Design review of the part built by this model. Coordinates are the model's own, in mm. Face numbers are marked on the shaded views. A direction names the side the tool comes from. Round coordinates to 2 decimals unless told otherwise and drop trailing zeros. Order: outer loops, then holes, each group sorted by start corner. A loop starts at its lowest first (then second) coordinate and runs counter-clockwise, first axis right, second up. Notation, with made-up numbers: M 58.5,-35 L 106.5,-35 A32 ccw 106.5,-3 Z; hole C 45,68.5 d6. An arc over 180 degrees is marked long. Use a Markdown table: item, result. Add a question column.
(1) To check wall thickness, follow probe 1 along Y at (x, z) = (-18, 111); probe 2 along Z at (x, y) = (-1.5, 2.5); probe 3 along X at (y, z) = (-0.5, 83). State the ranges of each line that lie inside material, in increasing order. Write a range as from..to.
(2) Take a section at A-A (y = 4.25). Write out the cut boundary in (x, z).
(3) For pin 1 (6 mm diameter, centred on x = -20.5, z = 105, fed in from +Y); pin 2 (5 mm diameter, centred on y = 0.5, z = 79, fed in from +X); pin 3 (0.7 mm diameter, centred on x = -0.07, y = 6.14, fed in from +Z); pin 4 (1.8 mm diameter, centred on y = 0, z = -1, fed in from +X), all flat-tipped, find the tip position at first contact; note any pin that passes through.
(4) Take a section at B-B (x = -9). Write out the cut boundary in (y, z).
(5) Machinability: for the marked faces 1 and 2, which of the approach directions +Z, -Z, +X, -X, +Y, -Y give a long, thin tool a straight path to every point of the face, cutting with its end or side? Answer none if there is none.
Autodesk Inventor part; units mm, degrees
ref_plane "YZ Plane" through (0, 0, 0) normal (1, 0, 0) x (0, 1, 0)
ref_plane "XZ Plane" through (0, 0, 0) normal (0, 1, 0) x (-1, 0, 0)
ref_plane "XY Plane" through (0, 0, 0) normal (0, 0, 1) x (1, 0, 0)
sketch "Sketch1" plane through (0, 0, 0) normal (0, 0, 1) x (1, 0, 0)
  line L0 (-6.698639, 7.691729) -> (4.001361, 7.691729)
  line L1 (4.001361, 7.691729) -> (4.001361, -6.308271)
  line L2 (4.001361, -6.308271) -> (-6.698639, -6.308271)
  line L3 (-6.698639, -6.308271) -> (-6.698639, 7.691729)
  line L4 (4.001361, -6.308271) -> (-6.698639, -6.308271)
  line L5 (-6.698639, -6.308271) -> (-6.698639, -2.808271)
  line L6 (-6.698639, -2.808271) -> (4.001361, -2.808271)
  line L7 (4.001361, -2.808271) -> (4.001361, -6.308271)
  line L8 (-6.698639, -6.308271) -> (-5.698639, -6.308271)
  line L9 (-5.698639, -6.308271) -> (-5.698639, 7.691729)
  line L10 (-5.698639, 7.691729) -> (-6.698639, 7.691729)
  line L11 (-6.698639, 7.691729) -> (-6.698639, -6.308271)
  line L12 (-5.698639, -2.808271) -> (3.472299, -2.808271)
  line L13 (3.472299, -2.808271) -> (3.472299, -0.408271)
  line L14 (3.472299, -0.408271) -> (-5.698639, -0.408271)
  line L15 (-5.698639, -0.408271) -> (-5.698639, -2.808271)
  line L16 (-5.698639, -0.408271) -> (-1.298639, -0.408271)
  line L17 (-1.298639, -0.408271) -> (-1.298639, -2.808271)
  line L18 (-1.298639, -2.808271) -> (-5.698639, -2.808271)
  line L19 (-5.698639, -2.808271) -> (-5.698639, -0.408271)
  point P0 (0, 0)
  dimension "d0" = 10.7
  dimension "d1" = 14
  dimension "d2" = 3.5
  dimension "d3" = 1
  dimension "d4" = 2.4
  dimension "d5" = 4.4
extrude "Extrusion1" add sketch "Sketch1" against normal blind 1.6
extrude "Extrusion2" add sketch "Sketch1" along normal blind 1.1 contours L14 L17 L6 L9
sketch "Sketch2" plane through (0, 0, 0) normal (0, 0, 1) x (1, 0, 0)
  line L0 (-1.298639, -0.408271) -> (-1.298639, -2.808271)
  line L1 (-1.298639, -2.808271) -> (-5.698639, -2.808271)
  line L2 (-5.698639, -2.808271) -> (-5.698639, -0.408271)
  line L3 (-5.698639, -0.408271) -> (-1.298639, -0.408271)
  line L4 (4.001361, 7.691729) -> (-6.698639, 7.691729)
  line L5 (-6.698639, 7.691729) -> (-6.698639, -6.308271)
  line L6 (-6.698639, -6.308271) -> (4.001361, -6.308271)
  line L7 (4.001361, -6.308271) -> (4.001361, 7.691729)
  line L8 (4.001361, -6.308271) -> (4.001361, 7.691729)
  line L9 (-6.698639, 7.691729) -> (-6.698639, -6.308271)
  line L10 (4.001361, -6.308271) -> (-6.698639, -6.308271)
  line L11 (-6.698639, -6.308271) -> (-6.698639, -5.308271)
  line L12 (-6.698639, -5.308271) -> (4.001361, -5.308271)
  line L13 (4.001361, -5.308271) -> (4.001361, -6.308271)
  line L14 (4.001361, -6.308271) -> (3.001361, -6.308271)
  line L15 (3.001361, -6.308271) -> (3.001361, -2.808271)
  line L16 (3.001361, -2.808271) -> (4.001361, -2.808271)
  line L17 (4.001361, -2.808271) -> (4.001361, -6.308271)
  line L18 (-6.698639, -6.308271) -> (-0.098639, -6.308271)
  line L19 (-0.098639, -6.308271) -> (-0.098639, -2.808271)
  line L20 (-0.098639, -2.808271) -> (-6.698639, -2.808271)
  line L21 (-6.698639, -2.808271) -> (-6.698639, -6.308271)
  circle A0 centre (1.451361, -3.758271) radius 1.55
  point P0 (0, 0)
  dimension "d10" = 1
  dimension "d11" = 1
  dimension "d12" = 6.6
extrude "Extrusion3" cut sketch "Sketch2" against normal through all contours A0
sketch "Sketch3" plane through (0, 0, 0) normal (0, 0, 1) x (1, 0, 0)
  line L0 (4.001361, 7.691729) -> (4.001361, -6.308271)
  line L1 (-6.698639, 7.691729) -> (4.001361, 7.691729)
  line L2 (4.001361, 7.691729) -> (4.001361, 6.691729)
  line L3 (4.001361, 6.691729) -> (-6.698639, 6.691729)
  line L4 (-6.698639, 6.691729) -> (-6.698639, 7.691729)
  line L5 (-6.698639, 7.691729) -> (-5.698639, 7.691729)
  line L6 (-5.698639, 7.691729) -> (-5.698639, 5.612457)
  line L7 (-5.698639, 5.612457) -> (-6.698639, 5.612457)
  line L8 (-6.698639, 5.612457) -> (-6.698639, 7.691729)
  line L9 (-5.698639, 6.691729) -> (-4.598639, 6.691729)
  line L10 (-4.598639, 6.691729) -> (-4.598639, 6.161753)
  line L11 (-4.598639, 6.161753) -> (-5.698639, 6.161753)
  line L12 (-5.698639, 6.161753) -> (-5.698639, 6.691729)
  circle A0 centre (-5.148639, 6.141729) radius 0.55
  circle A1 centre (-2.608639, 6.141729) radius 0.55
  line L13 (-2.058639, 6.161753) -> (-3.158639, 6.161753)
  circle A2 centre (-0.068639, 6.141729) radius 0.55
  line L14 (0.481361, 6.161753) -> (-0.618639, 6.161753)
  circle A3 centre (2.471361, 6.141729) radius 0.55
  line L15 (3.021361, 6.161753) -> (1.921361, 6.161753)
  circle A4 centre (1.451361, -3.758271) radius 1.55
  line L16 (-1.298639, -0.408271) -> (-1.298639, -2.808271)
  line L17 (-1.298639, -2.808271) -> (-5.698639, -2.808271)
  line L18 (-5.698639, -2.808271) -> (-5.698639, -0.408271)
  line L19 (-5.698639, -0.408271) -> (-1.298639, -0.408271)
  line L20 (4.001361, 7.691729) -> (-6.698639, 7.691729)
  line L21 (-6.698639, 7.691729) -> (-6.698639, -6.308271)
  line L22 (-6.698639, -6.308271) -> (4.001361, -6.308271)
  line L23 (4.001361, -6.308271) -> (4.001361, 7.691729)
  line L24 (-6.698639, -6.308271) -> (-5.698639, -6.308271)
  line L25 (-5.698639, -6.308271) -> (-5.698639, -3.371834)
  line L26 (-5.698639, -3.371834) -> (-6.698639, -3.371834)
  line L27 (-6.698639, -3.371834) -> (-6.698639, -6.308271)
  line L28 (-6.698639, -6.308271) -> (4.001361, -6.308271)
  line L29 (-6.698639, -6.308271) -> (-3.498639, -6.308271)
  line L30 (-3.498639, -6.308271) -> (-3.498639, -5.308271)
  line L31 (-3.498639, -5.308271) -> (-6.698639, -5.308271)
  line L32 (-6.698639, -5.308271) -> (-6.698639, -6.308271)
  line L33 (-5.698639, -6.308271) -> (-4.598639, -6.308271)
  line L34 (-4.598639, -6.308271) -> (-4.598639, -3.371834)
  line L35 (-4.598639, -3.371834) -> (-5.698639, -3.371834)
  line L36 (-5.698639, -3.371834) -> (-5.698639, -6.308271)
  circle A5 centre (-5.148639, -4.758271) radius 0.55
  circle A6 centre (-2.608639, -4.758271) radius 0.55
  line L37 (-0.958639, -5.308271) -> (-4.158639, -5.308271)
  point P0 (0, 0)
  dimension "d15" = 1
  dimension "d16" = 1
  dimension "d17" = 1.1
  dimension "d20" = 2.54
  dimension "d25" = 1
  dimension "d26" = 1
  dimension "d27" = 1.1
  dimension "d30" = 2.54
sketch "Sketch3 outline for Extrusion4" plane through (0, 0, 0) normal (0, 0, 1) x (1, 0, 0)
  circle A0 centre (-5.148639, -4.758271) radius 0.55
  circle A1 centre (-2.608639, -4.758271) radius 0.55
  circle A2 centre (2.471361, 6.141729) radius 0.55
  circle A3 centre (-0.068639, 6.141729) radius 0.55
  circle A4 centre (-2.608639, 6.141729) radius 0.55
  circle A5 centre (-5.148639, 6.141729) radius 0.55
extrude "Extrusion4" cut sketch "Sketch3 outline for Extrusion4" against normal through all
sketch "Sketch4" plane through (-5.698639, -0.408271, 0) normal (0, 1, 0) x (1, 0, 0)
  line L0 (0, 0) -> (4.4, 0)
  line L1 (0, 0) -> (0, -1.1)
  line L2 (4.4, -1.1) -> (0, -1.1)
  line L3 (4.4, 0) -> (4.4, -1.1)
  line L4 (0, -1.1) -> (4.4, -1.1)
  line L5 (2.2, -1.1) -> (2.2, 3.167795)
  line L6 (0, -1.1) -> (-26.909589, -122.481313)
  line L7 (0, -1.1) -> (4.299042, 18.291726)
  line L8 (4.4, -1.1) -> (31.309589, -122.481313)
  line L9 (4.4, -1.1) -> (0.100958, 18.291726)
  circle A0 centre (2.2, 8.823559) radius 134.49289
  point P0 (5.698639, 0)
  dimension "d37" = 12.5
extrude "Extrusion5" add sketch "Sketch4" against normal up to surface (2.4 mm away) contours L2 L8 A0 L6
sketch "Sketch5" plane through (-5.698639, -0.408271, 1.1) normal (-0.976296, 0, -0.2164396) x (-0.2164396, 0, 0.976296)
  line L0 (0, -2.4) -> (124.328392, -2.4)
  line L1 (124.328392, 0) -> (124.328392, -2.4)
  line L2 (0, 0) -> (124.328392, 0)
  line L3 (0, 0) -> (0, -2.4)
  line L4 (124.328392, 0) -> (124.328392, -2.4)
  line L5 (124.328392, 0) -> (111.727456, 0)
  line L6 (124.328392, -2.4) -> (123.022867, -2.4)
  line L7 (123.022867, -2.4) -> (123.022867, 0)
  line L8 (123.022867, 0) -> (124.328392, 0)
  line L9 (124.328392, 0) -> (124.328392, -2.4)
  point P0 (-2.307337, 0.408271)
  point P1 (123.022867, 0)
  point P2 (123.022867, -2.4)
extrude "Extrusion6" add sketch "Sketch5" along normal blind 1 contours L7 L2 L1 L0
sketch "Sketch6" plane through (25.610951, -0.408271, 122.481313) normal (0.976296, 0, -0.2164396) x (-0.2164396, 0, -0.976296)
  line L0 (0, -2.4) -> (124.328392, -2.4)
  line L1 (124.328392, -2.4) -> (124.328392, 0)
  line L2 (0, 0) -> (124.328392, 0)
  line L3 (0, 0) -> (0, -2.4)
  line L4 (0, 0) -> (0, -2.4)
  line L5 (0, -2.4) -> (124.328392, -2.4)
  line L6 (0, 0) -> (1.244112, 0)
  line L7 (1.244112, 0) -> (1.244112, -2.4)
  line L8 (1.244112, -2.4) -> (0, -2.4)
  line L9 (0, -2.4) -> (0, 0)
  point P0 (125.121241, 0.408271)
  point P1 (1.244112, -2.4)
  point P2 (1.244112, 0)
extrude "Extrusion7" add sketch "Sketch6" along normal blind 1 contours L3 L2 L7 L0
properties part number "TOF_VLCOS"
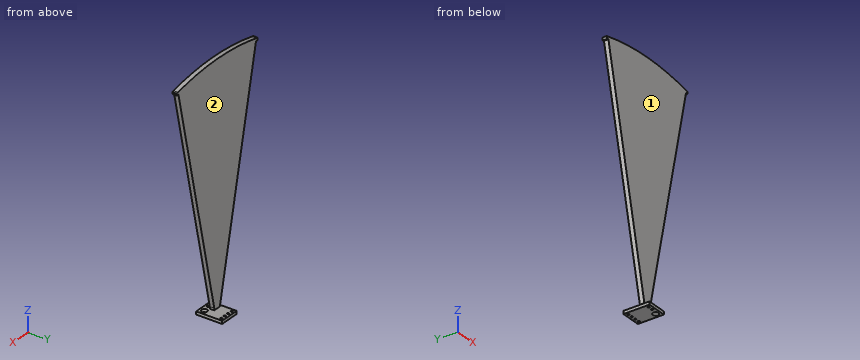
Verdict:
| question | item | result |
|---|---|---|
| 1 | probe 1 | y = -2.81..-0.41 |
| 1 | probe 2 | z = -1.6..0 |
| 1 | probe 3 | x = -23.86..16.86 |
| 2 | outline | M -6.7,-1.6 L 4,-1.6 L 4,0 L -6.7,0 Z |
| 3 | pin 1 | stops at y = -0.41 |
| 3 | pin 2 | stops at x = 16.49 |
| 3 | pin 3 | passes through |
| 3 | pin 4 | stops at x = 4 |
| 4 | outline | M -2.81,15.99 L -0.41,15.99 L -0.41,125.56 L -2.81,125.56 Z |
| 5 | face 1 | +Z, +X, -X, -Y |
| 5 | face 2 | +Z, +X, -X, +Y |
